The listing builds one solid part. Answer for the finished solid, in the listing's coordinates (mm). Face numbers are marked on the shaded views. Give positions to 0.01 mm unless a question says otherwise; leave off trailing zeros. Loops run counter-clockwise (first coordinate to the right, second up) from the corner with the lowest first, then second, coordinate; pieces in that order, holes last. Notation, with made-up numbers: (28, 56) - (39, 56) arc R25 ccw to (39, 75) - close; hole circle Ø2 at (-18.75, 22). An arc over 180 degrees is marked (long way). Answer as CSV lines item,"result". Start each with the question number.
1) A cutting plane is placed at D-D (z = -0.75). Determine the outline of the cut face in (x, y), and give its area (3 significant figures).
2) For a pull along X with two mould halves and no side action, classify the marked faces 1, 2, 3 and 4 as pulls with the +X half, pulls with the -X half, needs draft (parallel to the pull), parting line crosses it, or undercut.
3) Flat-ended cylindrical pins translate along their axes: pin 1 (3 mm diameter, centred on x = -3.5, z = 5.5, fed in from -Y); pin 2 (4 mm diameter, centred on x = 0, y = 1, fed in from +Z); pin 3 (5 mm diameter, centred on y = -5.5, z = 4, fed in from +X). Find the tip coordinate at first contact, or state that the pin passes through.
4) A cutting plane is placed at C-C (z = 5). Determine the outline of the cut face in (x, y), and give its area (3 significant figures).
5) Find the intervals of material crossed by line 1 along X through (y, z) = (0, 5.5); line 2 along Y through (x, z) = (0, -1.8); line 3 along Y through (x, z) = (0, -1.7), in increasing order.
6) A cutting plane is placed at A-A (x = 0). Determine the outline of the cut face in (y, z), and give its area (3 significant figures).
```python
from build123d import *

# Parameters (mm, degrees)
SKETCH4_R           = 18
SKETCH4_R_2         = 3.85
BOSS_EXTRUDE1_DEPTH = 8


with BuildPart() as part:
    # Sketch3 → Revolve2 (revolve)
    with BuildSketch(Plane(origin=(0, 0, 0), x_dir=(1, 0, 0), z_dir=(0, 1, 0))):
        with BuildLine():
            Line((0, 3.160044373), (3.85, 3.160044373))
            Line((3.85, 3.160044373), (3.85, 0))
            Line((3.85, 0), (18, 0))
            ThreePointArc((18, 0), (15.779795897, 3.046309242), (12.2, 1.865475811))
            Line((12.2, 1.865475811), (12.2, 1.74))
            Line((12.2, 1.74), (11.7, 1.74))
            Line((11.7, 1.74), (11.7, 2.2))
            Line((11.7, 2.2), (5, 2.2))
            Line((5, 2.2), (5, 1.61598722))
            Line((5, 1.61598722), (4.3, 1.61598722))
            Line((4.3, 1.61598722), (4.3, 3.376031593))
            ThreePointArc((4.3, 3.376031593), (2.194964612, 4.036754088), (0, 4.260044373))
            Line((0, 4.260044373), (0, 3.160044373))
        make_face()
    revolve(axis=Axis((0, 0, 0), (0, 0, -1)))

    # Sketch4 → Boss-Extrude1 (add)
    with BuildSketch(Plane.XY):
        Circle(SKETCH4_R)
        Circle(SKETCH4_R_2, mode=Mode.SUBTRACT)
    extrude(amount=BOSS_EXTRUDE1_DEPTH)


solid = part.part
```
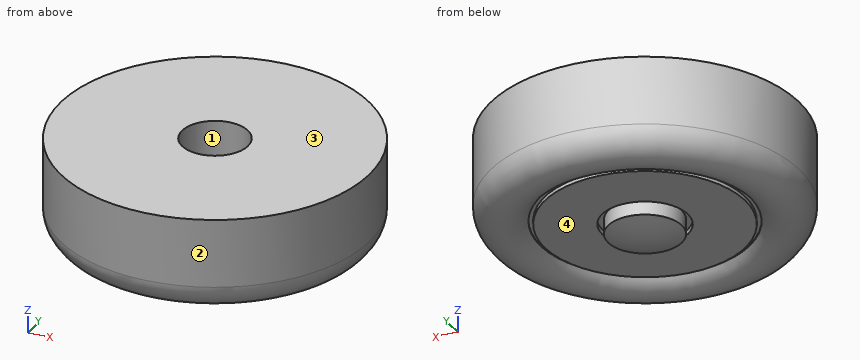
Ans:
1,outline,"circle Ø35.82 at (0, 0); hole circle Ø7.7 at (0, 0)"
1,area,"961 mm2"
2,face 1,"undercut"
2,face 2,"parting line crosses it"
2,face 3,"needs draft"
2,face 4,"undercut"
3,pin 1,"y = -17.89"
3,pin 2,"z = -3.16"
3,pin 3,"x = 17.75"
4,outline,"circle Ø36 at (0, 0); hole circle Ø7.7 at (0, 0)"
4,area,"971 mm2"
5,line 1,"-18 to -3.85, 3.85 to 18"
5,line 2,"-17.45 to -12.2, -11.7 to -5, -4.3 to -3.85, 3.85 to 4.3, 5 to 11.7, 12.2 to 17.45"
5,line 3,"-17.51 to -5, -4.3 to -3.85, 3.85 to 4.3, 5 to 17.51"
6,outline,"(-18, 0) arc R3.2 ccw to (-12.2, -1.87) - (-12.2, -1.74) - (-11.7, -1.74) - (-11.7, -2.2) - (-5, -2.2) - (-5, -1.62) - (-4.3, -1.62) - (-4.3, -3.38) arc R10.9 ccw to (4.3, -3.38) - (4.3, -1.62) - (5, -1.62) - (5, -2.2) - (11.7, -2.2) - (11.7, -1.74) - (12.2, -1.74) - (12.2, -1.87) arc R3.2 ccw to (18, 0) - (18, 8) - (3.85, 8) - (3.85, -3.16) - (-3.85, -3.16) - (-3.85, 8) - (-18, 8) - close"
6,area,"300 mm2"
